from build123d import *

# Parameters (mm, degrees)
SKETCH1_W           = 13
SKETCH1_H           = 60
BOSS_EXTRUDE1_DEPTH = 35
SKETCH3_W           = 1.5
SKETCH3_H           = 10
BOSS_EXTRUDE2_DEPTH = 1.5
SKETCH7_W           = 13.3
SKETCH7_H           = 17.5
SKETCH7_H_2         = 18
BOSS_EXTRUDE6_DEPTH = 35
SKETCH11_R          = 3.25
CUT_EXTRUDE2_DEPTH  = 27.3


with BuildPart() as part:
    # Sketch1 → Boss-Extrude1 (new body)
    with BuildSketch(Plane.XY):
        with Locations((6.5, 30)):
            Rectangle(SKETCH1_W, SKETCH1_H)
    extrude(amount=-BOSS_EXTRUDE1_DEPTH)

    # Sketch3 → Boss-Extrude2 (add)
    with BuildSketch(Plane(origin=(13, 0, 0), x_dir=(0, 0, -1), z_dir=(1, 0, 0))):
        with Locations((1.75, 30)):
            Rectangle(SKETCH3_W, SKETCH3_H)
    extrude(amount=BOSS_EXTRUDE2_DEPTH)

    # Sketch7 → Boss-Extrude6 (add)
    with BuildSketch(Plane.XY):
        with Locations((19.65, 51.25)):
            Rectangle(SKETCH7_W, SKETCH7_H)
        with Locations((19.65, 9)):
            Rectangle(SKETCH7_W, SKETCH7_H_2)
    extrude(amount=-BOSS_EXTRUDE6_DEPTH)

    # Sketch11 → Cut-Extrude2 (cut, through all)
    with BuildSketch(Plane(origin=(26.3, 0, 0), x_dir=(0, 0, -1), z_dir=(1, 0, 0))):
        with Locations((4.8, 4.8)):
            Circle(SKETCH11_R)
        with Locations((30.2, 4.8)):
            Circle(SKETCH11_R)
        with Locations((30.2, 55.6)):
            Circle(SKETCH11_R)
        with Locations((4.8, 55.6)):
            Circle(SKETCH11_R)
    extrude(amount=-CUT_EXTRUDE2_DEPTH, mode=Mode.SUBTRACT)


solid = part.part
Can you work these out from the model? Positions are in its coordinate system, mm. A direction names the side the tool comes from. Coordinates: 2 decimals unless noted, no trailing zeros. Order: outer loops, then holes, each group sorted by start corner. A loop starts at its lowest first (then second) coordinate and runs counter-clockwise, first axis right, second up. Notation, with made-up numbers: (18, 41) -> (62, 41) arc R27 cw to (62, 65) -> close; hole circle Ø5 at (-8, -15.5). An arc over 180 degrees is marked (long way). Use one line per item in the form item = value.
Q1. Imagine slicing it at B-B, the plane y = 4.8. List the corners of the cut face in (x, z) for me.
From the geometry:
outline = (0, -35) -> (26.3, -35) -> (26.3, -33.45) -> (0, -33.45) -> close; (0, -26.95) -> (26.3, -26.95) -> (26.3, -8.05) -> (0, -8.05) -> close; (0, -1.55) -> (26.3, -1.55) -> (26.3, 0) -> (0, 0) -> close
Q2. Imagine slicing it at C-C, the plane x = 19.5. List the corners of the cut face in (y, z) for me.
From the geometry:
outline = (0, -35) -> (18, -35) -> (18, 0) -> (0, 0) -> close; (42.5, -35) -> (60, -35) -> (60, 0) -> (42.5, 0) -> close; hole circle Ø6.5 at (4.8, -30.2); hole circle Ø6.5 at (4.8, -4.8); hole circle Ø6.5 at (55.6, -30.2); hole circle Ø6.5 at (55.6, -4.8)
Q3. Imagine slicing it at D-D, the plane x = 8.5. List the corners of the cut face in (y, z) for me.
From the geometry:
outline = (0, -35) -> (60, -35) -> (60, 0) -> (0, 0) -> close; hole circle Ø6.5 at (4.8, -30.2); hole circle Ø6.5 at (4.8, -4.8); hole circle Ø6.5 at (55.6, -30.2); hole circle Ø6.5 at (55.6, -4.8)
Q4. I need wall thicknesses on L1, parallel to Y at x = 18, z = -30.2; L2, parallel to Y at x = 1.75, z = -4.5; L3, parallel to Z at x = 16.75, y = 56.5. Which ranges of each line are inside material? Lowest first, please.
From the geometry:
L1 = 0 to 1.55, 8.05 to 18, 42.5 to 52.35, 58.85 to 60
L2 = 0 to 1.56, 8.04 to 52.36, 58.84 to 60
L3 = -35 to -33.32, -27.08 to -7.92, -1.68 to 0
Q5. Which directions (+Z, -Z, +X, -X, +Y, -Y) give clear straight access to the entire face, cutting with the end or side of a thin tool? Please do faces 1 (the face through (20, 18, -17)), 2 (the face through (0, 30, -17)), 3 (the face through (14, 30, -2.5)).
From the geometry:
face_1 = +Z, -Z, +X
face_2 = +Z, -Z, -X, +Y, -Y
face_3 = -Z, +X
Q6. We'd pull the mould along Y, two halves only. Please class faces 4 (the face through (13.33, 5.78, -7.9)), 5 (the face through (13, 0, -17)), 6 (the face through (10, 30, 0)): released by +Y, released by -Y, zero draft, split by the parting line, or undercut.
From the geometry:
face_4 = undercut
face_5 = released by -Y
face_6 = zero draft
Q7. Imagine slicing it at A-A, the plane z = -4.8. List the corners of the cut face in (x, y) for me.
From the geometry:
outline = (0, 0) -> (26.3, 0) -> (26.3, 1.55) -> (0, 1.55) -> close; (0, 8.05) -> (26.3, 8.05) -> (26.3, 18) -> (13, 18) -> (13, 42.5) -> (26.3, 42.5) -> (26.3, 52.35) -> (0, 52.35) -> close; (0, 58.85) -> (26.3, 58.85) -> (26.3, 60) -> (0, 60) -> close
Q8. Will these pins go through, and if not, where does the flat tip stop? P1, Ø1, axis at x = 3.5, y = 41, coming from the +Z side; P2, Ø0.8, axis at y = 32, z = -2, coming from the +X side; P3, Ø12, axis at y = 26, z = -11.5, coming from the +X side; P4, Ø0.8, axis at x = 13.5, y = 31, coming from the -Z side.
From the geometry:
P1 = 0
P2 = 14.5
P3 = 13
P4 = -2.5
